Could you check a few things on this model? Use its own coordinates, in mm. Round coordinates to 2 decimals unless told otherwise and drop trailing zeros. Write each loop counter-clockwise with the first axis right and the second up, starting at its lowest first coordinate (ties: lowest second). Pieces come first, ordered by that corner, then holes. Notation, with made-up numbers: (-39.75, -26) -> (6.25, -26) arc R28 cw to (6.25, 12) -> close; hole circle Ø8 at (79, 70.25). An arc over 180 degrees is marked (long way). Answer as CSV lines item,"result". Start each with the question number.
Q1. Will this pin go through, and if not, where does the flat tip stop? pin 1 Ø2 at (y, z) = (-1, 1) entering from -X.
Q2. Imagine slicing it at D-D on x = 9. Please give me the cut outline in (y, z).
Q3. If I drill on line 1 (X direction, y = -0.05, z = -0.05); line 2 (Y direction, x = 1.25, z = 1); line 3 (X direction, y = -1.55, z = 1.05), over which ranges is the centre line in solid material (lowest first)? Write a range as [from, to].
Q4. Imagine slicing it at C-C on z = -1.05. Please give me the cut outline in (x, y).
Q5. Imagine slicing it at A-A on x = 7.5. Please give me the cut outline in (y, z), and give its area (3 significant figures).
Q6. Imagine slicing it at B-B on y = 0. Please give me the cut outline in (x, z).
Autodesk Inventor part; units mm, degrees
ref_plane "Work Plane1" through (10, 0, 0) normal (1, 0, 0) x (0, 1, 0)
ref_plane "Work Plane2" through (10, 0, -10) normal (0.998, -0.0639, 0) x (0.0639, 0.998, 0)
ref_plane "YZ Plane" through (0, 0, 0) normal (1, 0, 0) x (0, 1, 0)
sketch "Skizze1" plane through (0, 0, 0) normal (0, 0, 1) x (1, 0, 0)
  line L0 (0, 0) -> (10, 0)
  line L1 (0.5, 2) -> (9.5, 2)
  arc A0 (0.5, 2) -> (0, 0) centre (4.25, 0) ccw
  arc A1 (10, 0) -> (9.5, 2) centre (5.75, 0) ccw
  line L2 (10, 0) -> (10, 1.68) construction
  line L3 (10, 1.68) -> (5, 2) construction
  line L4 (-12.8617, 0) -> (72.8617, 0)
  line L5 (0, 12.1847) -> (0, -2.0308)
  point P0 (5, 0)
  dimension "d0" = 4
  dimension "d1" = 10
  dimension "d2" = 3.36
  dimension "d12" = 5
  dimension "d17" = 0.5
  dimension "d18" = 0.5
revolve "Körper" add sketch "Skizze1" angle 360 about axis through (0, 0, 0) along (1, 0, 0)
ref_plane "Work Plane1" through (10, 0, 0) normal (1, 0, 0) x (0, 1, 0)
sketch "Skizze2" plane through (10, 0, 0) normal (1, 0, 0) x (0, 1, 0)
  line L0 (0, -14) -> (0, 14)
ref_plane "Work Plane2" through (10, 0, -10) normal (0.998, -0.0639, 0) x (0.0639, 0.998, 0)
sketch "Skizze3" plane through (10, 0, -10) normal (0.998, -0.0639, 0) x (0.0639, 0.998, 0)
  ellipse E0 centre (-0.0319, 10) end of major axis (-0.0319, 12) minor radius 1.9959
  line L0 (-0.3193, 10) -> (1.6766, 10)
  line L1 (1.6766, 10) -> (1.9545, 10.1946)
  line L2 (1.6766, 10) -> (1.9545, 9.8054)
  arc A0 (1.9545, 9.8054) -> (1.9545, 10.1946) centre (-0.0319, 10) ccw
  dimension "d7" = 70
extrude "Nut" cut sketch "Skizze3" against normal up to next contours L2 L1 E0 picked at (1.8643, 10.0973)
pattern_circular "Nuten" count 3 over 360 about axis through (5, 0, 0) along (1, 0, 0) of "Nut"
equation "\"d0\" = NND"
equation "\"d1\" = NLG"
equation "\"d2\" = 0.84 * NND"
equation "\"d18\" = KAH"
equation "\"d8\" = 0.5 * NLG"
equation "\"NND\" = 4"
equation "\"NLG\" = 10"
equation "\"KAH\" = 0.5"
equation "\"d6\" = -d5"
equation "\"FAC\" = 0.5"
equation "\"NND1\" = 4.25"
equation "\"NLG1\" = 9"
properties part number "ISO 8745 - 4 x 10" material "Edelstahl, austenitisch"
Checks:
1,pin 1,"x = 0.02"
2,outline,"(-1.15, -1.64) -> (-0.87, -1.51) -> (-0.85, -1.81) arc R2 ccw to (1.99, -0.17) -> (1.74, 0) -> (1.99, 0.17) arc R2 ccw to (-0.85, 1.81) -> (-0.87, 1.51) -> (-1.15, 1.64) arc R2 ccw to start"
3,line 1,"[0, 10]"
3,line 2,"[-1.73, 1.73]"
3,line 3,"[0.43, 9.57]"
4,outline,"(0.5, -1.7) -> (9.5, -1.7) arc R4.12 ccw to (9.5, 1.7) -> (0.5, 1.7) arc R4.12 ccw to start"
5,outline,"(-1.09, -1.67) -> (-0.92, -1.59) -> (-0.9, -1.78) arc R2 ccw to (2, -0.11) -> (1.84, 0) -> (2, 0.11) arc R2 ccw to (-0.9, 1.78) -> (-0.92, 1.59) -> (-1.09, 1.67) arc R2 ccw to start"
5,area,"12.5 mm^2"
6,outline,"(0.5, -2) -> (9.5, -2) arc R4.25 ccw to (9.5, 2) -> (0.5, 2) arc R4.25 ccw to start"
